from build123d import *

# Parameters (mm, degrees)
F0_W     = 114
F0_H     = 230
F1_DEPTH = 10


with BuildPart() as f1:
    # F0 (on Top) → F1 (new body)
    with BuildSketch(Plane.XY):
        with Locations((57, 115)):
            Rectangle(F0_W, F0_H)
        with BuildLine():
            Line((12, 32), (12, 198))
            ThreePointArc((12, 198), (17.857864, 212.142136), (32, 218))
            Line((32, 218), (82, 218))
            ThreePointArc((82, 218), (96.142136, 212.142136), (102, 198))
            Line((102, 198), (102, 50))
            ThreePointArc((102, 50), (96.142136, 35.857864), (82, 30))
            Line((82, 30), (74, 30))
            ThreePointArc((74, 30), (59.857864, 35.857864), (54, 50))
            Line((54, 50), (54, 200))
            Line((54, 200), (60, 200))
            Line((60, 200), (60, 50))
            ThreePointArc((60, 50), (64.100505, 40.100505), (74, 36))
            Line((74, 36), (82, 36))
            ThreePointArc((82, 36), (91.899495, 40.100505), (96, 50))
            Line((96, 50), (96, 198))
            ThreePointArc((96, 198), (91.899495, 207.899495), (82, 212))
            Line((82, 212), (32, 212))
            ThreePointArc((32, 212), (22.100505, 207.899495), (18, 198))
            Line((18, 198), (18, 32))
            ThreePointArc((18, 32), (22.100505, 22.100505), (32, 18))
            Line((32, 18), (102, 18))
            Line((102, 18), (102, 12))
            Line((102, 12), (82, 12))
            Line((82, 12), (32, 12))
            ThreePointArc((32, 12), (17.857864, 17.857864), (12, 32))
        make_face(mode=Mode.SUBTRACT)
    extrude(amount=F1_DEPTH)


solid = f1.part
Part model, mm, in its own coordinate system. A direction names the side the tool comes from. Give positions to 0.01 mm unless a question says otherwise; leave off trailing zeros. Loops run counter-clockwise (first coordinate to the right, second up) from the corner with the lowest first, then second, coordinate; pieces in that order, holes last.
(1) 3-axis set-ups, long thin cutter, end or side, ignore diameter. For faces 3 (the flat face through (102, 125, 5)), 4 (the flat face through (44, 117, 10)): which of +Z, -Z, +X, -X, +Y, -Y reach the whole face in a straight line?
Return value:
face 3: +Z, -Z
face 4: +Z, +X, -X, +Y, -Y
(2) Pull direction Y, two halves, no side cores. Call faces 1 (the flat face through (57, 212, 5)), 2 (the flat face through (0, 113, 5)): pulls with the +Y half, pulls with the -Y half, needs draft (parallel to the pull), parting line crosses it, or undercut.
Return value:
face 1: undercut
face 2: needs draft
(3) Band-saw the part on C-C (z = 7). Write the cut outline in (x, y).
Return value:
outline: (0, 0) - (114, 0) - (114, 230) - (0, 230) - close; hole (12, 32) arc R20 ccw to (32, 12) - (102, 12) - (102, 18) - (32, 18) arc R14 cw to (18, 32) - (18, 198) arc R14 cw to (32, 212) - (82, 212) arc R14 cw to (96, 198) - (96, 50) arc R14 cw to (82, 36) - (74, 36) arc R14 cw to (60, 50) - (60, 200) - (54, 200) - (54, 50) arc R20 ccw to (74, 30) - (82, 30) arc R20 ccw to (102, 50) - (102, 198) arc R20 ccw to (82, 218) - (32, 218) arc R20 ccw to (12, 198) - close
(4) Band-saw the part on D-D (y = 205). Write the cut outline in (x, z) (3 decimals).
Return value:
outline: (0, 0) - (13.265, 0) - (13.265, 10) - (0, 10) - close; (19.876, 0) - (94.124, 0) - (94.124, 10) - (19.876, 10) - close; (100.735, 0) - (114, 0) - (114, 10) - (100.735, 10) - close
(5) Band-saw the part on A-A (x = 40). Write the cut outline in (y, z).
Return value:
outline: (0, 0) - (12, 0) - (12, 10) - (0, 10) - close; (18, 0) - (212, 0) - (212, 10) - (18, 10) - close; (218, 0) - (230, 0) - (230, 10) - (218, 10) - close
(6) Drill centre lines: line 1 along Y through (x, z) = (47.5, 2); line 2 along X through (y, z) = (76.5, 0.5); line 3 along Y through (x, z) = (77.5, 9.25). Where is each one in solid material? Low to high.
Return value:
line 1: y = 0 to 12, 18 to 212, 218 to 230
line 2: x = 0 to 12, 18 to 54, 60 to 96, 102 to 114
line 3: y = 0 to 12, 18 to 30, 36 to 212, 218 to 230
(7) Pin check, flat tip, straight feed: pin 1 (5 mm diameter, centred on x = 58, z = 7, fed in from -Y). Stop position of the tip, or through.
Return value:
pin 1: stops at y = 0
(8) Band-saw the part on B-B (y = 83). Write the cut outline in (x, z), and give its area (3 significant figures).
Return value:
outline: (0, 0) - (12, 0) - (12, 10) - (0, 10) - close; (18, 0) - (54, 0) - (54, 10) - (18, 10) - close; (60, 0) - (96, 0) - (96, 10) - (60, 10) - close; (102, 0) - (114, 0) - (114, 10) - (102, 10) - close
area: 960 mm2
